Verification items for the finished model (mm, model axes). A direction names the side the tool comes from. Coordinates: 2 decimals unless noted, no trailing zeros. Order: outer loops, then holes, each group sorted by start corner. A loop starts at its lowest first (then second) coordinate and runs counter-clockwise, first axis right, second up. Notation, with made-up numbers: M 69.5,35 L 76.5,35 A20 cw 76.5,70 Z; hole C -9,-33.75 d3. An arc over 180 degrees is marked long. Return JSON: item names as keys, results as strings. Group by question number.
1. Gauge pin test, flat ends, axial feed: pin 1 (1.5 mm diameter, centred on x = -13, y = 21, fed in from +Z); pin 2 (3 mm diameter, centred on y = 7, z = 108, fed in from +X); pin 3 (3 mm diameter, centred on x = -8, z = 107.5, fed in from -Y). Record the tip position at first contact, or that the pin passes through.
2. Set-up check for faces 1 (the flat face through (11.3, 19.1, 0)), 2 (the flat face through (0, 0, 101.6)): record each of +Z, -Z, +X, -X, +Y, -Y from which the full face is reachable in a straight line by a thin tool's end or side.
3. Mould release check, pull along Y, two halves, no side actions. Record for faces 3 (the flat face through (0, 0, 127)), 4 (the cylindrical face through (-2.868, 21.847, 50.089)), 5 (the cylindrical face through (-30.133, 1.326, 82.283)): +Y half, -Y half, draft (parallel to the pull), parting line (faces both ways), or undercut.
4. Material ranges on line 1 along Y through (x, z) = (0, 67); line 2 along X through (y, z) = (-10.5, 96); line 3 along Y through (x, z) = (0, 41.5), recorded low to high.
5. Section check A-A, the plane z = 51. Record the cut outline in (x, y), plus the area to 3 significant figures.
6. Section check B-B, the plane z = 100. Record the cut outline in (x, y) (1 decimal), plus the area to 3 significant figures.
```python
from build123d import *

# Parameters (mm, degrees)
F0_R     = 30.1625
F1_DEPTH = 127
F2_R     = 25.4
F3_R     = 22.0345
F4_DEPTH = 101.6
F5_R     = 30.1625
F5_R_2   = 25.5905
F6_DEPTH = 63.5


with BuildPart() as f1:
    # F0 (on Top) → F1 (new body)
    with BuildSketch(Plane.XY):
        Circle(F0_R)
    extrude(amount=F1_DEPTH)

    # F2
    f2_edges = [f1.edges().sort_by_distance(p)[0] for p in [
        (-30.1625, 0, 127),
    ]]
    fillet(f2_edges, radius=F2_R)

    # F3 (on face) → F4 (cut)
    with BuildSketch(Plane.XY):
        Circle(F3_R)
    extrude(amount=F4_DEPTH, mode=Mode.SUBTRACT)

    # F5 (on face) → F6 (cut)
    with BuildSketch(Plane.XY):
        Circle(F5_R)
        Circle(F5_R_2, mode=Mode.SUBTRACT)
    extrude(amount=F6_DEPTH, mode=Mode.SUBTRACT)


solid = f1.part
```
Answers follow:
{
 "1": {"pin 1": "z = 118.25", "pin 2": "x = 28.99", "pin 3": "y = -28.88"},
 "2": {"face 1": "-Z, +X, -X, +Y, -Y", "face 2": "-Z"},
 "3": {"face 3": "draft", "face 4": "undercut", "face 5": "parting line"},
 "4": {"line 1": "-30.16 to -22.03, 22.03 to 30.16", "line 2": "-28.28 to -19.37, 19.37 to 28.28", "line 3": "-25.59 to -22.03, 22.03 to 25.59"},
 "5": {"outline": "C 0,0 d51.18; hole C 0,0 d44.07", "area": "532 mm^2"},
 "6": {"outline": "C 0,0 d60.3; hole C 0,0 d44.1", "area": "1,330 mm^2"}
}
